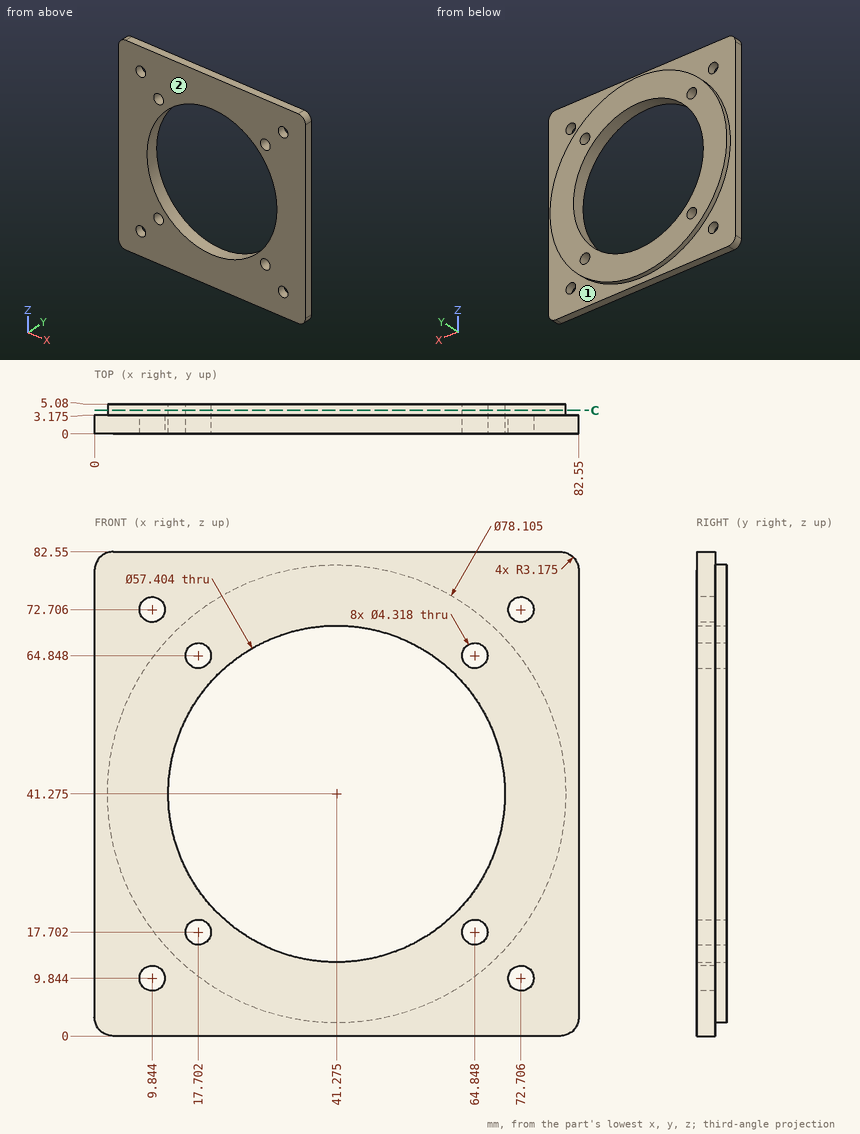
Job drawing, mm, ordinate dimensions from the low corner. One solid piece. A direction names the side the tool comes from. Give positions to 0.01 mm unless a question says otherwise; leave off trailing zeros. Order: outer loops, then holes, each group sorted by start corner. A loop starts at its lowest first (then second) coordinate and runs counter-clockwise, first axis right, second up. Notation, with made-up numbers: (57, 66.5) - (78, 66.5) arc R20 cw to (78, 98.5) - close; hole circle Ø11 at (72, 5.25). An arc over 180 degrees is marked (long way). Return JSON: item names as keys, results as strings.
1) Cut at C-C, the plane y = 4. Give the cut face in (x, z) (1 decimal), plus the area to 3 significant figures.
Geometry says:
{"outline": "circle Ø78.1 at (41.3, 41.3); hole circle Ø57.4 at (41.3, 41.3); hole circle Ø4.3 at (17.7, 17.7); hole circle Ø4.3 at (17.7, 64.8); hole circle Ø4.3 at (64.8, 17.7); hole circle Ø4.3 at (64.8, 64.8)", "area": "2,140 mm²"}
2) Flat gauge pins, fed straight in: P1, Ø3.5, axis at x = 72.71, z = 72.71, coming from the -Y side; P2, Ø5.5, axis at x = 64.85, z = 64.85, coming from the +Y side. Where does each tip first touch, or does it go through?
Geometry says:
{"P1": "through", "P2": "y = 5.08"}
3) Probe line 1 (X direction, y = 1.4, z = 10); line 2 (Z direction, x = 41, y = 2.35); line 3 (Z direction, x = 41, y = 3.4). List the from-to ranges inside material, lowest first. Write a range as from..to.
Geometry says:
{"line 1": "0..7.69, 12..70.55, 74.86..82.55", "line 2": "0..12.57, 69.98..82.55", "line 3": "2.22..12.57, 69.98..80.33"}
4) 3-axis set-ups, long thin cutter, end or side, ignore diameter. For the marked faces 1 and 2: which of +Z, -Z, +X, -X, +Y, -Y reach the whole face in a straight line?
Geometry says:
{"face 1": "+Y", "face 2": "+Z, -Z, +X, -X, -Y"}
